from build123d import *

# Parameters (mm, degrees)
F0_R     = 3.25
F0_R_2   = 1.65
F1_DEPTH = 7.5
F2_R     = 5.25
F2_R_2   = 3.25
F3_DEPTH = 25


# Not quite as in the source:
# - a fillet or chamfer that OpenCascade refuses, or shapes differently, is made with other operations: its cross-section is extruded or revolved along the edge and cut away or added


with BuildPart() as f1:
    # F0 (on Front) → F1 (new body)
    with BuildSketch(Plane.XZ):
        with BuildLine():
            Line((-3, 30), (-6.4811743939, 37.693775202))
            Line((-6.4811743939, 37.693775202), (-4.9623487879, 25.387550404))
            ThreePointArc((-4.9623487879, 25.387550404), (-4.6009153843, 27.9574416023), (-3, 30))
        make_face()
        with BuildLine():
            Line((4.9623487879, 25.387550404), (6.4811743939, 37.693775202))
            Line((6.4811743939, 37.693775202), (3, 30))
            ThreePointArc((3, 30), (4.472135955, 28.2360679775), (5, 26))
            ThreePointArc((5, 26), (4.9905783202, 25.6931970822), (4.9623487879, 25.387550404))
        make_face()
        with BuildLine():
            Line((-28.5, 0), (-23.5, -5))
            Line((-23.5, -5), (23.5, -5))
            Line((23.5, -5), (28.5, 0))
            Line((28.5, 0), (28.5, 26))
            Line((28.5, 26), (38, 35.8959565787))
            Line((38, 35.8959565787), (38, 50))
            Line((38, 50), (32, 50))
            Line((32, 50), (32, 40))
            Line((32, 40), (14, 40))
            Line((14, 40), (14, 50))
            Line((14, 50), (8, 50))
            Line((8, 50), (6.4811743939, 37.693775202))
            Line((6.4811743939, 37.693775202), (4.9623487879, 25.387550404))
            ThreePointArc((4.9623487879, 25.387550404), (0, 21), (-4.9623487879, 25.387550404))
            Line((-4.9623487879, 25.387550404), (-6.4811743939, 37.693775202))
            Line((-6.4811743939, 37.693775202), (-8, 50))
            Line((-8, 50), (-14, 50))
            Line((-14, 50), (-14, 40))
            Line((-14, 40), (-32, 40))
            Line((-32, 40), (-32, 50))
            Line((-32, 50), (-38, 50))
            Line((-38, 50), (-38, 35.8959565787))
            Line((-38, 35.8959565787), (-28.5, 26))
            Line((-28.5, 26), (-28.5, 0))
        make_face()
        with Locations((-17.25, 6.25)):
            Circle(F0_R, mode=Mode.SUBTRACT)
        with Locations((0, 3)):
            Circle(F0_R_2, mode=Mode.SUBTRACT)
        with Locations((17.25, 6.25)):
            Circle(F0_R, mode=Mode.SUBTRACT)
        with Locations((0, 14.3)):
            Circle(F0_R_2, mode=Mode.SUBTRACT)
    extrude(amount=F1_DEPTH)

    # F2 (on face) → F3 (join)
    with BuildSketch(Plane.XZ.offset(7.5)):
        with Locations((-17.25, 6.25)):
            Circle(F2_R)
        with Locations((-17.25, 6.25)):
            Circle(F2_R_2, mode=Mode.SUBTRACT)
        with Locations((17.25, 6.25)):
            Circle(F2_R)
        with Locations((17.25, 6.25)):
            Circle(F2_R_2, mode=Mode.SUBTRACT)
    extrude(amount=F3_DEPTH)

    # F4: fillet of radius 5 on 4 edges, made by hand

    # F4_s1 → F4_t2 (revolve)
    with BuildSketch(Plane.XY.offset(6.25)):
        with BuildLine():
            ThreePointArc((-7, -7.5), (-10.5355339059, -8.9644660941), (-12, -12.5))
            Line((-12, -12.5), (-12, -7.5))
            Line((-12, -7.5), (-7, -7.5))
        make_face()
    revolve(axis=Axis((-17.25, -7.5, 6.25), (0, -1, 0)))

    # F4_s3 → F4_t4 (revolve)
    with BuildSketch(Plane.XY.offset(6.25)):
        with BuildLine():
            ThreePointArc((27.5, -7.5), (23.9644660941, -8.9644660941), (22.5, -12.5))
            Line((22.5, -12.5), (22.5, -7.5))
            Line((22.5, -7.5), (27.5, -7.5))
        make_face()
    revolve(axis=Axis((17.25, -7.5, 6.25), (0, -1, 0)))

    # F4_s5 → F4_t6 (revolve, cut)
    with BuildSketch(Plane.XY.offset(6.25)):
        with BuildLine():
            ThreePointArc((20.5, -28.5), (21.027864045, -30.7360679775), (22.5, -32.5))
            Line((22.5, -32.5), (20.5, -32.5))
            Line((20.5, -32.5), (20.5, -28.5))
        make_face()
    revolve(axis=Axis((17.25, -32.5, 6.25), (0, -1, 0)), mode=Mode.SUBTRACT)

    # F4_s7 → F4_t8 (revolve, cut)
    with BuildSketch(Plane.XY.offset(6.25)):
        with BuildLine():
            ThreePointArc((-14, -28.5), (-13.472135955, -30.7360679775), (-12, -32.5))
            Line((-12, -32.5), (-14, -32.5))
            Line((-14, -32.5), (-14, -28.5))
        make_face()
    revolve(axis=Axis((-17.25, -32.5, 6.25), (0, -1, 0)), mode=Mode.SUBTRACT)


solid = f1.part
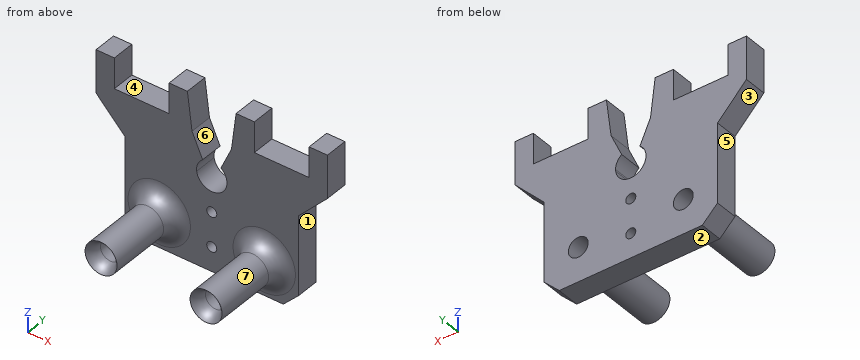
Build history of the part. All positions in model axes, mm. Face numbers are marked on the shaded views. A direction names the side the tool comes from. Round coordinates to 2 decimals unless told otherwise and drop trailing zeros. Write each loop counter-clockwise with the first axis right and the second up, starting at its lowest first coordinate (ties: lowest second). Pieces come first, ordered by that corner, then holes. Notation, with made-up numbers: (-20.5, -31.5) - (-16.5, -31.5) arc R26 cw to (-16.5, -4.5) - close; hole circle Ø4 at (-27.75, 64.25). An arc over 180 degrees is marked (long way). One line per question, with ' | ' between items.
1. Band-saw the part on B-B, the plane z = 6.25. Write the cut outline in (x, y), and give its area (3 significant figures).
Results are:
outline: (-28.5, -7.5) - (-27.5, -7.5) arc R5 cw to (-22.5, -12.5) - (-22.5, -32.5) arc R5 ccw to (-20.5, -28.5) - (-20.5, 0) - (-28.5, 0) - close; (-14, -28.5) arc R5 ccw to (-12, -32.5) - (-12, -12.5) arc R5 cw to (-7, -7.5) - (7, -7.5) arc R5 cw to (12, -12.5) - (12, -32.5) arc R5 ccw to (14, -28.5) - (14, 0) - (-14, 0) - close; (20.5, -28.5) arc R5 ccw to (22.5, -32.5) - (22.5, -12.5) arc R5 cw to (27.5, -7.5) - (28.5, -7.5) - (28.5, 0) - (20.5, 0) - close | area: 542 mm^2
2. Drill centre lines: line 1 along Z through (x, y) = (0, -1.5); line 2 along X through (y, z) = (-20.5, 8.5); line 3 along Z through (x, y) = (-17.25, -22.25). Where is each one in solid material? Low to high. Write a range as from..to.
Results are:
line 1: -5..1.35, 4.65..12.65, 15.95..21 | line 2: -21.99..-19.6, -14.9..-12.51, 12.51..14.9, 19.6..21.99 | line 3: 1..3, 9.5..11.5
3. Band-saw the part on D-D, the plane y = -18. Write the cut outline in (x, z).
Results are:
outline: circle Ø10.5 at (-17.25, 6.25); circle Ø10.5 at (17.25, 6.25); hole circle Ø6.5 at (-17.25, 6.25); hole circle Ø6.5 at (17.25, 6.25)
4. Drop flat-ended pins along their axis: pin 1 Ø5 at (x, z) = (16, 27) entering from -Y; pin 2 Ø4 at (y, z) = (-2, 9.5) entering from +X; pin 3 Ø6 at (x, y) = (27, -3.5) entering from +Z. Give the stop position or say it passes through.
Results are:
pin 1: y = -7.5 | pin 2: x = 28.5 | pin 3: z = 40
5. Band-saw the part on C-C, the plane y = -2. Write the cut outline in (x, z).
Results are:
outline: (-38, 35.9) - (-28.5, 26) - (-28.5, 0) - (-23.5, -5) - (23.5, -5) - (28.5, 0) - (28.5, 26) - (38, 35.9) - (38, 50) - (32, 50) - (32, 40) - (14, 40) - (14, 50) - (8, 50) - (6.48, 37.69) - (3, 30) arc R5 cw (long way) to (-3, 30) - (-6.48, 37.69) - (-8, 50) - (-14, 50) - (-14, 40) - (-32, 40) - (-32, 50) - (-38, 50) - close; hole circle Ø6.5 at (-17.25, 6.25); hole circle Ø3.3 at (0, 3); hole circle Ø3.3 at (0, 14.3); hole circle Ø6.5 at (17.25, 6.25)
6. Mould opens along X. For the marked faces 1, 2, 3 and 4 say: released by +X, released by -X, zero draft, split by the parting line, or undercut.
Results are:
face 1: released by +X | face 2: zero draft | face 3: released by -X | face 4: undercut
7. Tool access for the marked faces 5, 6 and 7: list every direction of +Z, -Z, +X, -X, +Y, -Y with a clear straight run to the whole face (end or side of a thin tool).
Results are:
face 5: -Z, -X, +Y, -Y | face 6: +Z, +Y, -Y | face 7: -Y
8. Band-saw the part on A-A, the plane x = 17.25. Write the cut outline in (y, z), and give its area (3 significant figures).
Results are:
outline: (-32.5, 1) - (-12.5, 1) arc R5 cw to (-7.5, -4) - (-7.5, -5) - (0, -5) - (0, 3) - (-28.5, 3) arc R5 ccw to start; (-32.5, 11.5) arc R5 ccw to (-28.5, 9.5) - (0, 9.5) - (0, 40) - (-7.5, 40) - (-7.5, 16.5) arc R5 cw to (-12.5, 11.5) - close | area: 395 mm^2
